Could you check a few things on this model? Use its own coordinates, in mm. A direction names the side the tool comes from. Give positions to 0.01 mm unless a question says otherwise; leave off trailing zeros. Order: outer loops, then holes, each group sorted by start corner. A loop starts at its lowest first (then second) coordinate and runs counter-clockwise, first axis right, second up. Notation, with made-up numbers: (33.25, -4.5) -> (57.25, -4.5) arc R20 ccw to (57.25, 10.5) -> close; hole circle Ø5 at (55.25, -14.75). An arc over 180 degrees is marked (long way). Write each question's results on one line, items separated by ' | '.
```python
from build123d import *

# Parameters (mm, degrees)
SKETCH2_W           = 32.91869007
SKETCH2_H           = 44.826135242
BOSS_EXTRUDE1_DEPTH = 10
SKETCH3_R           = 6
BOSS_EXTRUDE2_DEPTH = 10
SKETCH4_R           = 3
BOSS_EXTRUDE3_DEPTH = 10


with BuildPart() as part:
    # Sketch2 → Boss-Extrude1 (new body)
    with BuildSketch(Plane.XY):
        Rectangle(SKETCH2_W, SKETCH2_H)
    extrude(amount=BOSS_EXTRUDE1_DEPTH)

    # Sketch3 → Boss-Extrude2 (add)
    with BuildSketch(Plane.XY.offset(10)):
        Circle(SKETCH3_R)
    extrude(amount=BOSS_EXTRUDE2_DEPTH)

    # Sketch4 → Boss-Extrude3 (add)
    with BuildSketch(Plane.XY.offset(20)):
        Circle(SKETCH4_R)
    extrude(amount=BOSS_EXTRUDE3_DEPTH)


solid = part.part
```
Q1. Suppose I cut it at C-C on z = 15. Please give me the cut outline in (x, y), and give its area (3 significant figures).
Here are the results:
outline: circle Ø12 at (0, 0) | area: 113 mm²
Q2. Suppose I cut it at D-D on y = 9. Please give me the cut outline in (x, z), and give its area (3 significant figures).
Here are the results:
outline: (-16.46, 0) -> (16.46, 0) -> (16.46, 10) -> (-16.46, 10) -> close | area: 329 mm²
Q3. I'm going to push flat-ended pins straight in: pin 1 Ø6 at (x, z) = (-1.5, 20.5) entering from -Y; pin 2 Ø10 at (y, z) = (4.5, 12) entering from -X; pin 3 Ø4 at (x, y) = (6.5, -1) entering from +Z; pin 4 Ø12 at (x, z) = (-11.5, 18.5) entering from -Y. Where does each tip first touch, or does it pass through?
Here are the results:
pin 1: stops at y = -6 | pin 2: stops at x = -16.46 | pin 3: stops at z = 20 | pin 4: stops at y = -2.4
Q4. For faces 1 (the flat face through (-4, 5, 10)), 2 (the flat face through (-16.459, 0, 5)), which set-ups out of +Z, -Z, +X, -X, +Y, -Y let a thin tool reach every point of the face, with its end or its side?
Here are the results:
face 1: +Z | face 2: +Z, -Z, -X, +Y, -Y
Q5. Suppose I cut it at A-A on y = 0. Please give me the cut outline in (x, z).
Here are the results:
outline: (-16.46, 0) -> (16.46, 0) -> (16.46, 10) -> (6, 10) -> (6, 20) -> (3, 20) -> (3, 30) -> (-3, 30) -> (-3, 20) -> (-6, 20) -> (-6, 10) -> (-16.46, 10) -> close
Q6. I need wall thicknesses on line 1 along Z through (x, y) = (2, 9.5); line 2 along Z through (x, y) = (-3.5, 2); line 3 along X through (y, z) = (-1, 23.25). Which ranges of each line are inside material? Lowest first, please.
Here are the results:
line 1: z = 0 to 10 | line 2: z = 0 to 20 | line 3: x = -2.83 to 2.83
Q7. Suppose I cut it at B-B on x = 0. Please give me the cut outline in (y, z), and give its area (3 significant figures).
Here are the results:
outline: (-22.41, 0) -> (22.41, 0) -> (22.41, 10) -> (6, 10) -> (6, 20) -> (3, 20) -> (3, 30) -> (-3, 30) -> (-3, 20) -> (-6, 20) -> (-6, 10) -> (-22.41, 10) -> close | area: 628 mm²
